Verification items for this drawing (mm, ordinates from the low corner). Coordinates: 2 decimals unless noted, no trailing zeros. Write each loop counter-clockwise with the first axis right and the second up, starting at its lowest first coordinate (ties: lowest second). Pieces come first, ordered by that corner, then holes. Notation, with made-up numbers: M 28.5,57 L 59.5,57 A29 ccw 59.5,92 Z; hole C 57,-11 d7. An arc over 180 degrees is marked long. Put each result on its own line as item: value. Start each with the question number.
1) Cross-section at A-A on y = 1.7. Record the cut outline in (x, z), plus the area to 3 significant figures.
2) Cross-section at C-C on z = 51. Record the cut outline in (x, y), plus the area to 3 significant figures.
3) Cross-section at B-B on x = 109.5. Record the cut outline in (y, z), plus the area to 3 significant figures.
4) Scan lines: line 1 along Z through (x, y) = (185.2, 0.6); line 2 along X through (y, z) = (1.3, 100); line 3 along Z through (x, y) = (121, 2.4). Record each from-to range of solid material in increasing order.
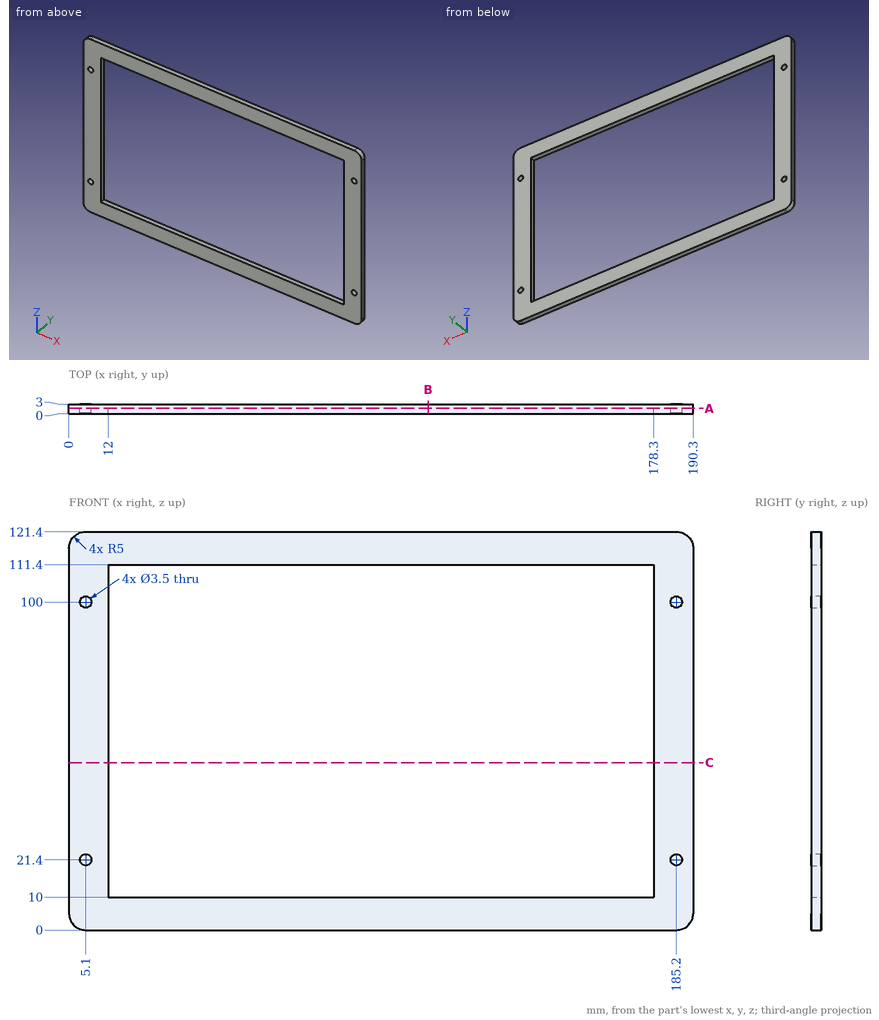
Answer key:
1. outline: M 0,5 A5 ccw 5,0 L 185.3,0 A5 ccw 190.3,5 L 190.3,116.4 A5 ccw 185.3,121.4 L 5,121.4 A5 ccw 0,116.4 Z; hole C 5.1,21.4 d3.5; hole C 5.1,100 d3.5; hole M 12,10 L 178.3,10 L 178.3,111.4 L 12,111.4 Z; hole C 185.2,21.4 d3.5; hole C 185.2,100 d3.5
1. area: 6,180 mm²
2. outline: M 0,0 L 12,0 L 12,3 L 0,3 Z; M 178.3,0 L 190.3,0 L 190.3,3 L 178.3,3 Z
2. area: 72.0 mm²
3. outline: M 0,0 L 3,0 L 3,10 L 0,10 Z; M 0,111.4 L 3,111.4 L 3,121.4 L 0,121.4 Z
3. area: 60.0 mm²
4. line 1: z = 0 to 19.65, 23.15 to 98.25, 101.75 to 121.4
4. line 2: x = 0 to 3.35, 6.85 to 12, 178.3 to 183.45, 186.95 to 190.3
4. line 3: z = 0 to 10, 111.4 to 121.4
